Geometry: see drawing. Coordinates: mm, zero at the bounding-box minimum. Round coordinates to 2 decimals unless told otherwise and drop trailing zeros. Order: outer loops, then holes, each group sorted by start corner. A loop starts at its lowest first (then second) coordinate and runs counter-clockwise, first axis right, second up. Notation, with made-up numbers: (-30.5, 85.5) -> (22.5, 85.5) arc R15 ccw to (22.5, 95.5) -> close; hole circle Ø1 at (-26.75, 77). An arc over 180 degrees is marked (long way). Answer as CSV lines item,"result". Start each with the question number.
(1) Section query A-A (y = 0.15). Output: boundary loops of the cut face in (x, z).
(2) Section query B-B (x = 86.5). Output: boundary loops of the cut face in (y, z), plus the area to 3 significant figures.
(3) Contact query for flat-ended pins moving along their axis: P1, Ø5, axis at x = 16.5, z = 55, coming from the -Y side; P2, Ø0.5, axis at y = 0.5, z = 42, coming from the -X side. Output: stop coordinate, or through.
(4) Section query C-C (z = 44). Output: boundary loops of the cut face in (x, y).
(5) Line query: line 1 along Z through (x, y) = (19.5, 0.1); line 2 along Z through (x, y) = (57, 0.1); line 3 along X through (y, z) = (0.35, 34). Output: solid intervals per line, ascending. Write a range as from..to.
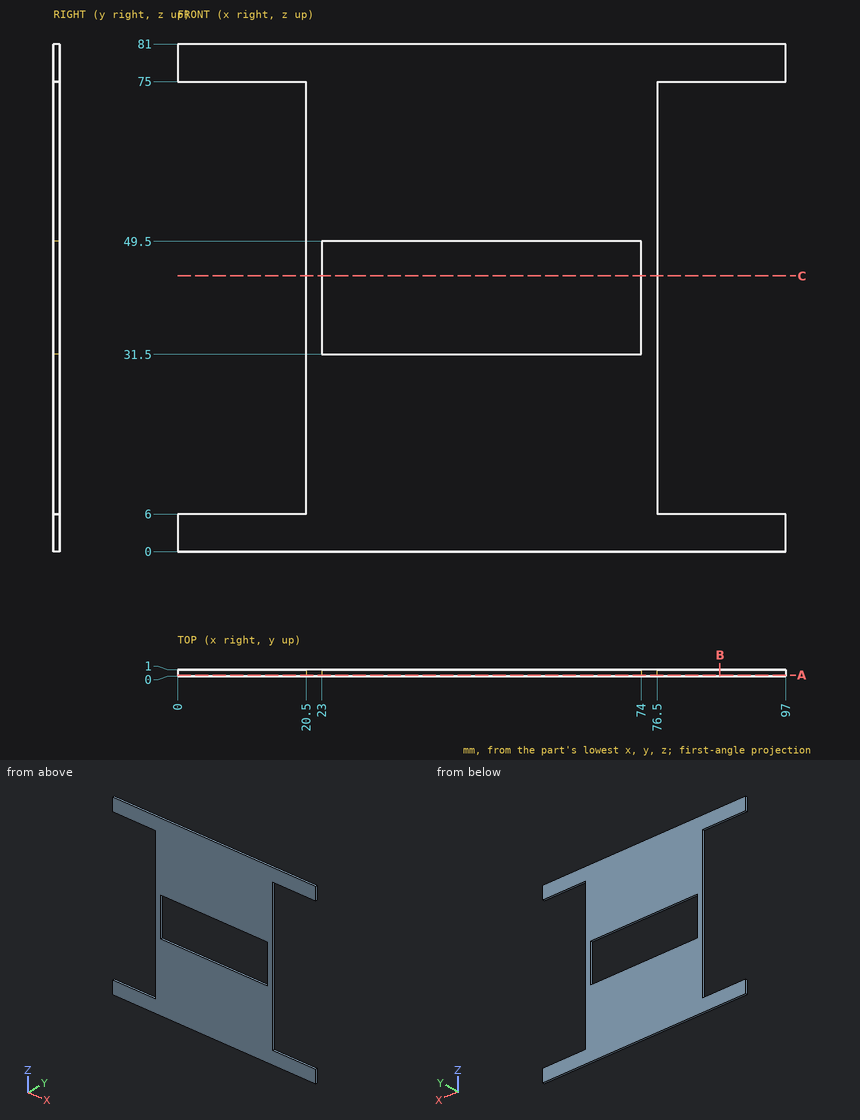
Answer block:
1,outline,"(0, 0) -> (97, 0) -> (97, 6) -> (76.5, 6) -> (76.5, 75) -> (97, 75) -> (97, 81) -> (0, 81) -> (0, 75) -> (20.5, 75) -> (20.5, 6) -> (0, 6) -> close; hole (23, 31.5) -> (74, 31.5) -> (74, 49.5) -> (23, 49.5) -> close"
2,outline,"(0, 0) -> (1, 0) -> (1, 6) -> (0, 6) -> close; (0, 75) -> (1, 75) -> (1, 81) -> (0, 81) -> close"
2,area,"12.0 mm2"
3,P1,"through"
3,P2,"x = 20.5"
4,outline,"(20.5, 0) -> (23, 0) -> (23, 1) -> (20.5, 1) -> close; (74, 0) -> (76.5, 0) -> (76.5, 1) -> (74, 1) -> close"
5,line 1,"0..6, 75..81"
5,line 2,"0..31.5, 49.5..81"
5,line 3,"20.5..23, 74..76.5"
